Could you check a few things on this model? Use its own coordinates, in mm. Face numbers are marked on the shaded views. A direction names the side the tool comes from. Give positions to 0.01 mm unless a question says otherwise; leave off trailing zeros. Loops run counter-clockwise (first coordinate to the right, second up) from the corner with the lowest first, then second, coordinate; pieces in that order, holes last. Notation, with made-up numbers: (55, 70.25) - (101, 70.25) arc R15 cw to (101, 87.25) - close; hole circle Ø3 at (1, 23). An arc over 180 degrees is marked (long way). Answer in a Markdown table with one row per item. Add a question column.
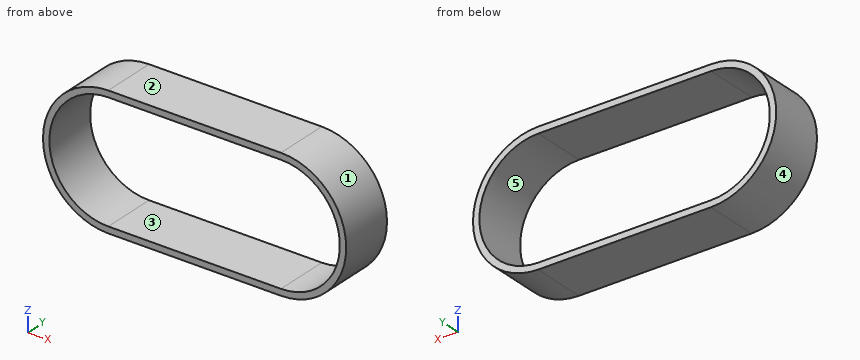
```python
from build123d import *

# Parameters (mm, degrees)
PAD_DEPTH = 7.5


with BuildPart() as part:
    # Sketch → Pad (new body, symmetric)
    with BuildSketch(Plane.XZ):
        with BuildLine():
            ThreePointArc((0, 18), (-18, 0), (0, -18))
            Line((0, -18), (47.6, -18))
            ThreePointArc((47.6, -18), (65.6, 0), (47.6, 18))
            Line((0, 18), (47.6, 18))
        make_face()
        with BuildLine():
            ThreePointArc((0, 16.25), (-16.25, 0), (0, -16.25))
            Line((0, -16.25), (47.6, -16.25))
            ThreePointArc((47.6, -16.25), (63.85, 0), (47.6, 16.25))
            Line((0, 16.25), (47.6, 16.25))
        make_face(mode=Mode.SUBTRACT)
    extrude(amount=PAD_DEPTH, both=True)


solid = part.part
```
(1) Please list where these lines run through material, in increasing order: line 1 (Z direction, x = 30.5, y = 3.75); line 2 (X direction, y = -2.75, z = 0); line 3 (Z direction, x = 58, y = 4.25).
(2) I want a section at A-A on x = 43. Please give me the cut outline in (y, z).
(3) I want a section at C-C on y = 5.5. Please give me the cut outline in (x, z).
(4) We'd pull the mould along X, two halves only. Please class the marked faces 1, 2 and 3: pulls with the +X half, pulls with the -X half, needs draft (parallel to the pull), parting line crosses it, or undercut.
(5) I want a section at B-B on z = 0. Please give me the cut outline in (x, y), then the cut area to 3 significant figures.
(6) On a 3-axis mill with a long thin cutter (end or side, diameter ignored), from which of +Z, -Z, +X, -X, +Y, -Y can I reach the whole of each face in a straight line? I mean the marked faces 4 and 5. Say none if no direction works.
(7) For pin 1 Ø8 at (y, z) = (4.5, 5.5) entering from +X; pin 2 Ø1 at (x, y) = (54.5, 0.5) entering from -Z; pin 3 Ø3 at (x, y) = (49.5, -1.5) entering from +Z, each with a flat end and sliding along its axis, tell me the tip position at first contact or that it passes through.
Reported:
| question | item | result |
|---|---|---|
| 1 | line 1 | -18 to -16.25, 16.25 to 18 |
| 1 | line 2 | -18 to -16.25, 63.85 to 65.6 |
| 1 | line 3 | -14.69 to -12.49, 12.49 to 14.69 |
| 2 | outline | (-7.5, -18) - (7.5, -18) - (7.5, -16.25) - (-7.5, -16.25) - close; (-7.5, 16.25) - (7.5, 16.25) - (7.5, 18) - (-7.5, 18) - close |
| 3 | outline | (0, -18) - (47.6, -18) arc R18 ccw to (47.6, 18) - (0, 18) arc R18 ccw to start; hole (0, -16.25) - (47.6, -16.25) arc R16.25 ccw to (47.6, 16.25) - (0, 16.25) arc R16.25 ccw to start |
| 4 | face 1 | pulls with the +X half |
| 4 | face 2 | needs draft |
| 4 | face 3 | undercut |
| 5 | outline | (-18, -7.5) - (-16.25, -7.5) - (-16.25, 7.5) - (-18, 7.5) - close; (63.85, -7.5) - (65.6, -7.5) - (65.6, 7.5) - (63.85, 7.5) - close |
| 5 | area | 52.5 mm² |
| 6 | face 4 | -X, +Y, -Y |
| 6 | face 5 | +Y, -Y |
| 7 | pin 1 | x = 65.54 |
| 7 | pin 2 | z = -16.82 |
| 7 | pin 3 | z = 18 |
